```python
from build123d import *

# Parameters (mm, degrees)
SKETCH1_R           = 3.686275202
SKETCH1_R_2         = 1.5
BOSS_EXTRUDE1_DEPTH = 10
CUT_SWEEP1_ANGLE    = 65.162978
SKETCH3_R           = 2
SKETCH4_R           = 2
SKETCH5_R           = 2
CUT_SWEEP5_ANGLE    = 66.926183


# Read off the part's stored shape, not the designer's step: Cut-Sweep1, Cut-Sweep5
with BuildPart() as part:
    # Sketch1 → Boss-Extrude1 (new body)
    with BuildSketch(Plane.XY):
        with BuildLine():
            Line((49.491190341, 2.55078162), (63.988368206, 3.929851578))
            ThreePointArc((63.988368206, 3.929851578), (68.649398374, 10.07494702), (69.613421186, 17.727270865))
            Line((69.613421186, 17.727270865), (69.514351105, 17.71366502))
            ThreePointArc((69.514351105, 17.71366502), (66.543133225, 24.775071071), (60.439280034, 29.404819157))
            Line((60.439280034, 29.404819157), (60.363775967, 29.219618898))
            ThreePointArc((60.363775967, 29.219618898), (52.865525757, 30.164231855), (45.899544112, 27.233165568))
            Line((45.899544112, 27.233165568), (46.022180208, 27.075176998))
            ThreePointArc((46.022180208, 27.075176998), (41.517560448, 21.136292813), (40.585887394, 13.740758359))
            Line((40.585887394, 13.740758359), (40.784027557, 13.767970048))
            ThreePointArc((40.784027557, 13.767970048), (43.634790659, 6.992837216), (49.491190341, 2.55078162))
        make_face()
        with Locations((56.226488574, 8.636175254)):
            Circle(SKETCH1_R, mode=Mode.SUBTRACT)
        with Locations((54.851979087, 15.7)):
            Circle(SKETCH1_R_2, mode=Mode.SUBTRACT)
    extrude(amount=-BOSS_EXTRUDE1_DEPTH)

    # Cut-Sweep1 outline → Cut-Sweep1 (revolve, cut)
    with BuildSketch(Plane(origin=(54.851979087, 15.7, 0), x_dir=(0.5396064408716191, -0.8419173884472655, 0), z_dir=(-0.8419173884472655, -0.5396064408716191, 0))):
        with BuildLine():
            Line((14.9, -6.5612495), (14.9, -3.4387505))
            ThreePointArc((14.9, -3.4387505), (14.15, -5), (14.9, -6.5612495))
        make_face()
    revolve(axis=Axis((54.851979087, 15.7, 0), (0, 0, 1)), revolution_arc=CUT_SWEEP1_ANGLE, mode=Mode.SUBTRACT)

    # Cut-Sweep2: sweep along a curve in space
    with BuildLine() as cut_sweep2_path:
        ThreePointArc((69.514351105, 17.71366502, 0), (66.543133225, 24.775071071, 0), (60.439280034, 29.404819157, 0))
    # Sketch3 → Cut-Sweep2 (sweep, cut)
    with BuildSketch(Plane(origin=(41.545913318, -16.937802546, 0), x_dir=(0, 0, 1), z_dir=(-0.9260012944005722, 0.37752033424501136, 0))):
        with Locations((-5, 51.295957801)):
            Circle(SKETCH3_R)
    sweep(path=cut_sweep2_path.line, mode=Mode.SUBTRACT)

    # Cut-Sweep3: sweep along a curve in space
    with BuildLine() as cut_sweep3_path:
        ThreePointArc((60.363775967, 29.219618898, 0), (52.865525757, 30.164231855, 0), (45.899544112, 27.233165568, 0))
    # Sketch4 → Cut-Sweep3 (sweep, cut)
    with BuildSketch(Plane(origin=(41.832894366, 32.472113961, 0), x_dir=(0, 0, 1), z_dir=(-0.7899428471017035, -0.6131804777656041, 0))):
        with Locations((-5, -5.382060044)):
            Circle(SKETCH4_R)
    sweep(path=cut_sweep3_path.line, mode=Mode.SUBTRACT)

    # Cut-Sweep4: sweep along a curve in space
    with BuildLine() as cut_sweep4_path:
        ThreePointArc((46.022180208, 27.075176998, 0), (41.517560448, 21.136292813, 0), (40.585887394, 13.740758359, 0))
    # Sketch5 → Cut-Sweep4 (sweep, cut)
    with BuildSketch(Plane(origin=(-1.100839052, 8.015688586, 0), x_dir=(0.9907008120106874, 0.13605844729881716, 0), z_dir=(0.13605844729881716, -0.9907008120106874, 0))):
        with Locations((40.828017845, -5)):
            Circle(SKETCH5_R)
    sweep(path=cut_sweep4_path.line, mode=Mode.SUBTRACT)

    # Cut-Sweep5 outline → Cut-Sweep5 (revolve, cut)
    with BuildSketch(Plane(origin=(54.851979087, 15.7, 0), x_dir=(-0.9907008120106691, -0.13605844729894895, 0), z_dir=(-0.13605844729894895, 0.9907008120106691, 0))):
        with BuildLine():
            ThreePointArc((14.20000016, -3.438750372), (13.45, -5.000000221), (14.200000505, -6.561249904))
            Line((14.200000505, -6.561249904), (14.20000016, -3.438750372))
        make_face()
    revolve(axis=Axis((54.851979087, 15.7, 0), (0, 0, 1)), revolution_arc=CUT_SWEEP5_ANGLE, mode=Mode.SUBTRACT)


solid = part.part
```
Input: part model. Units: mm. Frame: model coordinates. Coordinates: 2 decimals unless noted, no trailing zeros. Loops run counter-clockwise (first coordinate to the right, second up) from the corner with the lowest first, then second, coordinate; pieces in that order, holes last. Notation, with made-up numbers: M 48.25,86 L 55.25,86 A29 cw 55.25,113 Z; hole C -15.5,-7.75 d3. An arc over 180 degrees is marked long. Use a Markdown table: item, result. Add a question column.
1) Section A-A, the plane z = -7.25. Return the cut outline in (x, y).
2) Draft query along X for faces 1 (the cylindrical face through (41.558, 21.234, -1.695)), 2 (the cylindrical face through (68.608, 9.974, -1.695)), 3 (the cylindrical face through (52.544, 8.798, -4.93)). Return one class per face: +X half, -X half, draft (parallel to the pull), parting line (faces both ways), or undercut.
3) Pin query (flat end, axial travel): P1, Ø5, axis at x = 51, y = 22.5, coming from the +Z side; P2, Ø1, axis at y = 20.5, z = -2, coming from the +X side; P3, Ø4, axis at y = 7.5, z = -5, coming from the +X side. Return the tip coordinate at first contact, or that it passes through.
4) Line query: L1, parallel to X at y = 14.5, z = -9; L2, parallel to Y at x = 58, z = -0.5; L3, parallel to X at y = 11.25, z = -5.5. Output: solid intervals per line, ascending. Write a range as from..to.
Answer below:
| question | item | result |
|---|---|---|
| 1 | outline | M 40.59,13.74 L 40.78,13.77 A14.2 ccw 49.49,2.55 L 63.99,3.93 A14.9 ccw 69.61,17.73 L 69.51,17.71 A14.8 ccw 60.44,29.4 L 60.36,29.22 A14.6 ccw 45.9,27.23 L 46.02,27.08 A14.4 ccw Z; hole C 56.23,8.64 d7.37; hole C 54.85,15.7 d3 |
| 2 | face 1 | -X half |
| 2 | face 2 | +X half |
| 2 | face 3 | undercut |
| 3 | P1 | z = 0 |
| 3 | P2 | x = 69.01 |
| 3 | P3 | x = 68.03 |
| 4 | L1 | 40.5..53.95, 55.75..69.7 |
| 4 | L2 | 3.36..5.4, 11.87..29.96 |
| 4 | L3 | 42.09..53.63, 58.83..68.35 |
